from build123d import *

# Parameters (mm, degrees)
SKETCH1_W           = 124
SKETCH1_H           = 68
BOSS_EXTRUDE1_DEPTH = 12
SKETCH2_W           = 120
SKETCH2_H           = 64
CUT_EXTRUDE1_DEPTH  = 10
FILLET1_R           = 0.5


with BuildPart() as part:
    # Sketch1 → Boss-Extrude1 (new body)
    with BuildSketch(Plane(origin=(0, 0, 0), x_dir=(1, 0, 0), z_dir=(0, 1, 0))):
        with Locations((62, 34)):
            Rectangle(SKETCH1_W, SKETCH1_H)
    extrude(amount=BOSS_EXTRUDE1_DEPTH)

    # Sketch2 → Cut-Extrude1 (cut)
    with BuildSketch(Plane(origin=(0, 12, 0), x_dir=(1, 0, 0), z_dir=(0, 1, 0))):
        with Locations((62, 34)):
            Rectangle(SKETCH2_W, SKETCH2_H)
    extrude(amount=-CUT_EXTRUDE1_DEPTH, mode=Mode.SUBTRACT)

    # Fillet1
    fillet1_edges = [part.edges().sort_by_distance(p)[0] for p in [
        (124, 12, -34),
        (62, 12, -68),
        (62, 2, -66),
        (2, 7, -66),
        (122, 2, -34),
        (122, 7, -66),
        (62, 2, -2),
        (122, 7, -2),
        (2, 2, -34),
        (2, 7, -2),
        (62, 12, -66),
        (2, 12, -34),
        (62, 12, -2),
        (122, 12, -34),
        (0, 12, -34),
        (62, 0, -68),
        (124, 0, -34),
        (62, 0, 0),
        (0, 0, -34),
        (62, 12, 0),
        (0, 6, -68),
        (124, 6, -68),
        (124, 6, 0),
        (0, 6, 0),
    ]]
    fillet(fillet1_edges, radius=FILLET1_R)


solid = part.part
Geometry: final body of the model. Coordinates: model frame, mm. A direction names the side the tool comes from. Round coordinates to 2 decimals unless told otherwise and drop trailing zeros. Loops run counter-clockwise (first coordinate to the right, second up) from the corner with the lowest first, then second, coordinate; pieces in that order, holes last.
Q1. Pull-direction query (X, two-part tool) for faces 3 (the flat face through (0, 6, -34)), 4 (the flat face through (61, 0, -34)), 5 (the flat face through (61, 7, -66)); classes: released by +X, released by -X, zero draft, split by the parting line, or undercut.
Q2. Pin query (flat end, axial travel): P1, Ø1, axis at x = 96.5, z = -43.5, coming from the +Y side; P2, Ø7, axis at x = 53.5, y = 9, coming from the +Z side. Return the tip coordinate at first contact, or that it passes through.
Q3. Material intervals for L1, parallel to X at y = 6.75, z = -26; L2, parallel to Z at x = 98.5, y = 3.5; L3, parallel to Y at x = 32, z = -47, sorted ascending.
Q4. Section A-A on y = 5. Return loops of the section in (x, z), plus the area to 3 significant figures.
Q5. Section B-B on z = -20.5. Return loops of the section in (x, y), plus the area to 3 significant figures.
Q6. Section C-C on x = 8. Return loops of the section in (y, z), plus the area to 3 significant figures.
Q7. Access query for faces 1 (the flat face through (61, 6, -68)), 2 (the flat face through (122, 7, -34)). Directions: +Z, -Z, +X, -X, +Y, -Y. A direction counts if a zero-diameter tool reaches every point of the face in a straight line with its end or side. Return the directions, or none.
Evaluation:
1. face 3: released by -X
1. face 4: zero draft
1. face 5: undercut
2. P1: stops at y = 2
2. P2: stops at z = 0
3. L1: x = 0 to 2, 122 to 124
3. L2: z = -68 to -66, -2 to 0
3. L3: y = 0 to 2
4. outline: (0, -67.5) arc R0.5 ccw to (0.5, -68) - (123.5, -68) arc R0.5 ccw to (124, -67.5) - (124, -0.5) arc R0.5 ccw to (123.5, 0) - (0.5, 0) arc R0.5 ccw to (0, -0.5) - close; hole (2, -65.5) arc R0.5 ccw to (2.5, -66) - (121.5, -66) arc R0.5 ccw to (122, -65.5) - (122, -2.5) arc R0.5 ccw to (121.5, -2) - (2.5, -2) arc R0.5 ccw to (2, -2.5) - close
4. area: 752 mm2
5. outline: (0, 0.5) arc R0.5 ccw to (0.5, 0) - (123.5, 0) arc R0.5 ccw to (124, 0.5) - (124, 11.5) arc R0.5 ccw to (123.5, 12) - (122.5, 12) arc R0.5 ccw to (122, 11.5) - (122, 2.5) arc R0.5 cw to (121.5, 2) - (2.5, 2) arc R0.5 cw to (2, 2.5) - (2, 11.5) arc R0.5 ccw to (1.5, 12) - (0.5, 12) arc R0.5 ccw to (0, 11.5) - close
5. area: 288 mm2
6. outline: (0, -67.5) arc R0.5 ccw to (0.5, -68) - (11.5, -68) arc R0.5 ccw to (12, -67.5) - (12, -66.5) arc R0.5 ccw to (11.5, -66) - (2.5, -66) arc R0.5 cw to (2, -65.5) - (2, -2.5) arc R0.5 cw to (2.5, -2) - (11.5, -2) arc R0.5 ccw to (12, -1.5) - (12, -0.5) arc R0.5 ccw to (11.5, 0) - (0.5, 0) arc R0.5 ccw to (0, -0.5) - close
6. area: 176 mm2
7. face 1: -Z, +X, -X, +Y, -Y
7. face 2: +Y
